from build123d import *

# Parameters (mm, degrees)
SKETCH_1_W          = 30
SKETCH_1_H          = 40
SKETCH_1_W_2        = 28
SKETCH_1_H_2        = 38
EXTRUDE_1_DEPTH     = 90
SKETCH_2_R          = 1.55
CUT_EXTRUDE_1_DEPTH = 40
SKETCH_3_R          = 2.1
CUT_EXTRUDE_2_DEPTH = 10
SKETCH_4_R          = 15
CUT_EXTRUDE_3_DEPTH = 40
SKETCH_5_R          = 2.1
SKETCH_5_R_2        = 1.6
CUT_EXTRUDE_4_DEPTH = 10
SKETCH_6_R          = 4
CUT_EXTRUDE_5_DEPTH = 10
CUT_EXTRUDE_START   = -50
SKETCH_7_R          = 2.1
CUT_EXTRUDE_6_DEPTH = 50


with BuildPart() as part:
    # 草图1 → 凸台-拉伸1 (new, symmetric)
    with BuildSketch(Plane.XY):
        Rectangle(SKETCH_1_W, SKETCH_1_H)
        Rectangle(SKETCH_1_W_2, SKETCH_1_H_2, mode=Mode.SUBTRACT)
    extrude(amount=EXTRUDE_1_DEPTH, both=True)

    # 草图2 → 切除-拉伸1 (cut, symmetric)
    with BuildSketch(Plane(origin=(0, 20, 0), x_dir=(1, 0, 0), z_dir=(0, 1, 0))):
        with Locations(Location((-8, -84, 0), (0, 0, 270))):
            Circle(SKETCH_2_R)
        with Locations(Location((8, -84, 0), (0, 0, 270))):
            Circle(SKETCH_2_R)
        with Locations(Location((8, -66, 0), (0, 0, 270))):
            Circle(SKETCH_2_R)
        with Locations(Location((-8, -66, 0), (0, 0, 270))):
            Circle(SKETCH_2_R)
        with Locations(Location((-8, 66, 0), (0, 0, 270))):
            Circle(SKETCH_2_R)
        with Locations(Location((8, 66, 0), (0, 0, 270))):
            Circle(SKETCH_2_R)
        with Locations(Location((8, 84, 0), (0, 0, 270))):
            Circle(SKETCH_2_R)
        with Locations(Location((-8, 84, 0), (0, 0, 270))):
            Circle(SKETCH_2_R)
    extrude(amount=CUT_EXTRUDE_1_DEPTH, both=True, mode=Mode.SUBTRACT)

    # 草图3 → 切除-拉伸2 (cut)
    with BuildSketch(Plane(origin=(0, -19, 0), x_dir=(1, 0, 0), z_dir=(0, 1, 0))):
        with Locations(Location((5, -55.51, 0), (0, 0, 270))):
            Circle(SKETCH_3_R)
        with Locations(Location((5, -18.51, 0), (0, 0, 270))):
            Circle(SKETCH_3_R)
        with Locations(Location((5, 18.49, 0), (0, 0, 270))):
            Circle(SKETCH_3_R)
        with Locations(Location((5, 55.49, 0), (0, 0, 270))):
            Circle(SKETCH_3_R)
    extrude(amount=-CUT_EXTRUDE_2_DEPTH, mode=Mode.SUBTRACT)

    # 草图4 → 切除-拉伸3 (cut)
    with BuildSketch(Plane.ZY.offset(15)):
        with Locations(Location((18.5, 0, 0), (0, 0, 270))):
            Circle(SKETCH_4_R)
        with Locations(Location((-18.5, 0, 0), (0, 0, 180))):
            Circle(SKETCH_4_R)
        with BuildLine():
            Line((63, 13), (69, 13))
            ThreePointArc((69, 13), (76.071067812, 10.071067812), (79, 3))
            Line((79, 3), (79, -3))
            ThreePointArc((79, -3), (76.071067812, -10.071067812), (69, -13))
            Line((69, -13), (63, -13))
            ThreePointArc((63, -13), (55.928932188, -10.071067812), (53, -3))
            Line((53, -3), (53, 3))
            ThreePointArc((53, 3), (55.928932188, 10.071067812), (63, 13))
        make_face()
        with BuildLine():
            Line((-63, -13), (-69, -13))
            ThreePointArc((-69, -13), (-76.071067812, -10.071067812), (-79, -3))
            Line((-79, -3), (-79, 3))
            ThreePointArc((-79, 3), (-76.071067812, 10.071067812), (-69, 13))
            Line((-69, 13), (-63, 13))
            ThreePointArc((-63, 13), (-55.928932188, 10.071067812), (-53, 3))
            Line((-53, 3), (-53, -3))
            ThreePointArc((-53, -3), (-55.928932188, -10.071067812), (-63, -13))
        make_face()
    extrude(amount=-CUT_EXTRUDE_3_DEPTH, mode=Mode.SUBTRACT)

    # 草图5 → 切除-拉伸4 (cut)
    with BuildSketch(Plane(origin=(0, 20, 0), x_dir=(1, 0, 0), z_dir=(0, 1, 0))):
        with Locations(Location((-8, 0, 0), (0, 0, 270))):
            Circle(SKETCH_5_R)
        with Locations(Location((-8, 12.5, 0), (0, 0, 270))):
            Circle(SKETCH_5_R_2)
        with Locations(Location((-8, -12.5, 0), (0, 0, 270))):
            Circle(SKETCH_5_R_2)
    extrude(amount=-CUT_EXTRUDE_4_DEPTH, mode=Mode.SUBTRACT)

    # 草图6 → 切除-拉伸5 (cut)
    with BuildSketch(Plane(origin=(0, -19, 0), x_dir=(1, 0, 0), z_dir=(0, 1, 0))):
        with Locations(Location((-8, -12.5, 0), (0, 0, 270))):
            Circle(SKETCH_6_R)
        with Locations(Location((-8, 12.5, 0), (0, 0, 270))):
            Circle(SKETCH_6_R)
        with Locations(Location((-8, 0, 0), (0, 0, 270))):
            Circle(SKETCH_6_R)
    extrude(amount=-CUT_EXTRUDE_5_DEPTH, mode=Mode.SUBTRACT)

    # 草图7 → 切除-拉伸6 (cut)
    with BuildSketch(Plane.XZ.offset(20).offset(CUT_EXTRUDE_START)):
        with Locations(Location((5, -55.49, 0), (0, 0, 90))):
            Circle(SKETCH_7_R)
        with Locations(Location((5, -18.49, 0), (0, 0, 90))):
            Circle(SKETCH_7_R)
        with Locations(Location((5, 18.51, 0), (0, 0, 90))):
            Circle(SKETCH_7_R)
        with Locations(Location((5, 55.51, 0), (0, 0, 90))):
            Circle(SKETCH_7_R)
    extrude(amount=CUT_EXTRUDE_6_DEPTH, mode=Mode.SUBTRACT)


solid = part.part
The listing builds one solid part. Answer for the finished solid, in the listing's coordinates (mm). A direction names the side the tool comes from. Round coordinates to 2 decimals unless told otherwise and drop trailing zeros. Loops run counter-clockwise (first coordinate to the right, second up) from the corner with the lowest first, then second, coordinate; pieces in that order, holes last. Notation, with made-up numbers: M -19,19.25 L 23,19.25 A33 cw 23,51.25 Z; hole C 87.5,24 d8. An arc over 180 degrees is marked long. Return JSON: item names as keys, results as strings.
Q1. Which of the six approach directions +Z, -Z, +X, -X, +Y, -Y give full straight-line access (tool end or side, diameter ignored) to faces 1 (the face through (0, -19, 1)), 2 (the face through (-14.51, -9.99, -55.85)), 3 (the face through (-10.4, -19.5, -3.2))?
Results list:
{"face 1": "+Z, -Z", "face 2": "+X, -X", "face 3": "-Y"}
Q2. Find the intervals of material crossed by line 1 along X through (y, z) = (-19.65, -84); line 2 along Y through (x, z) = (9.25, 50); line 3 along X through (y, z) = (-1, 46.5), in increasing order. Write a range as from..to.
Results list:
{"line 1": "x = -15..-9.55, -6.45..6.45, 9.55..15", "line 2": "y = -20..-19, 19..20", "line 3": "x = -15..-14, 14..15"}
Q3. Find section C-C, the plane x = 11.5. Determine the outline of the cut face in (y, z).
Results list:
{"outline": "M -20,-90 L -19,-90 L -19,90 L -20,90 Z; M 19,-90 L 20,-90 L 20,90 L 19,90 Z"}
Q4. Find section D-D, the plane z = 84. Determine the outline of the cut face in (x, y), plus the area to 3 significant figures.
Results list:
{"outline": "M -15,-20 L -9.55,-20 L -9.55,-19 L -14,-19 L -14,19 L -9.55,19 L -9.55,20 L -15,20 Z; M -6.45,-20 L 6.45,-20 L 6.45,-19 L -6.45,-19 Z; M -6.45,19 L 6.45,19 L 6.45,20 L -6.45,20 Z; M 9.55,-20 L 15,-20 L 15,20 L 9.55,20 L 9.55,19 L 14,19 L 14,-19 L 9.55,-19 Z", "area": "124 mm2"}
Q5. Find section A-A, the plane z = 0. Determine the outline of the cut face in (x, y).
Results list:
{"outline": "M -15,-20 L -12,-20 L -12,-19 L -14,-19 L -14,19 L -10.1,19 L -10.1,20 L -15,20 Z; M -5.9,19 L 14,19 L 14,-19 L -4,-19 L -4,-20 L 15,-20 L 15,20 L -5.9,20 Z"}
Q6. The mould has two halves that part along X. Classify faces 4 (the face through (14.493, 3.252, 3.857)), 5 (the face through (6.278, 19.507, -57.156)): released by +X, released by -X, zero draft, split by the parting line, or undercut.
Results list:
{"face 4": "zero draft", "face 5": "undercut"}
Q7. This flat-tipped pin is pushed along its axis until it touches: pin 1 Ø1.5 at (y, z) = (1, -4) entering from -X. Where does it stop, or does it pass through?
Results list:
{"pin 1": "stops at x = -15"}
Q8. Find section B-B, the plane z = -66. State how many separate pieces and enclosed holes the cut face has, plus the area to 3 significant figures.
Results list:
{"separate pieces": "6", "enclosed holes": "0", "area": "71.6 mm2"}
